The drawing under review shows one solid part. Ordinate dimensions are in mm from its lowest x, y, z. A direction names the side the tool comes from. Give positions to 0.01 mm unless a question says otherwise; leave off trailing zeros. Write each loop counter-clockwise with the first axis right and the second up, starting at its lowest first coordinate (ties: lowest second). Pieces come first, ordered by that corner, then holes. Notation, with made-up numbers: (69, -7.5) - (76, -7.5) arc R25 ccw to (76, 22.5) - close; hole circle Ø10 at (-1.75, -9). An arc over 180 degrees is marked (long way). Write each question's results on one line, items separated by ' | '. Start each with the question number.
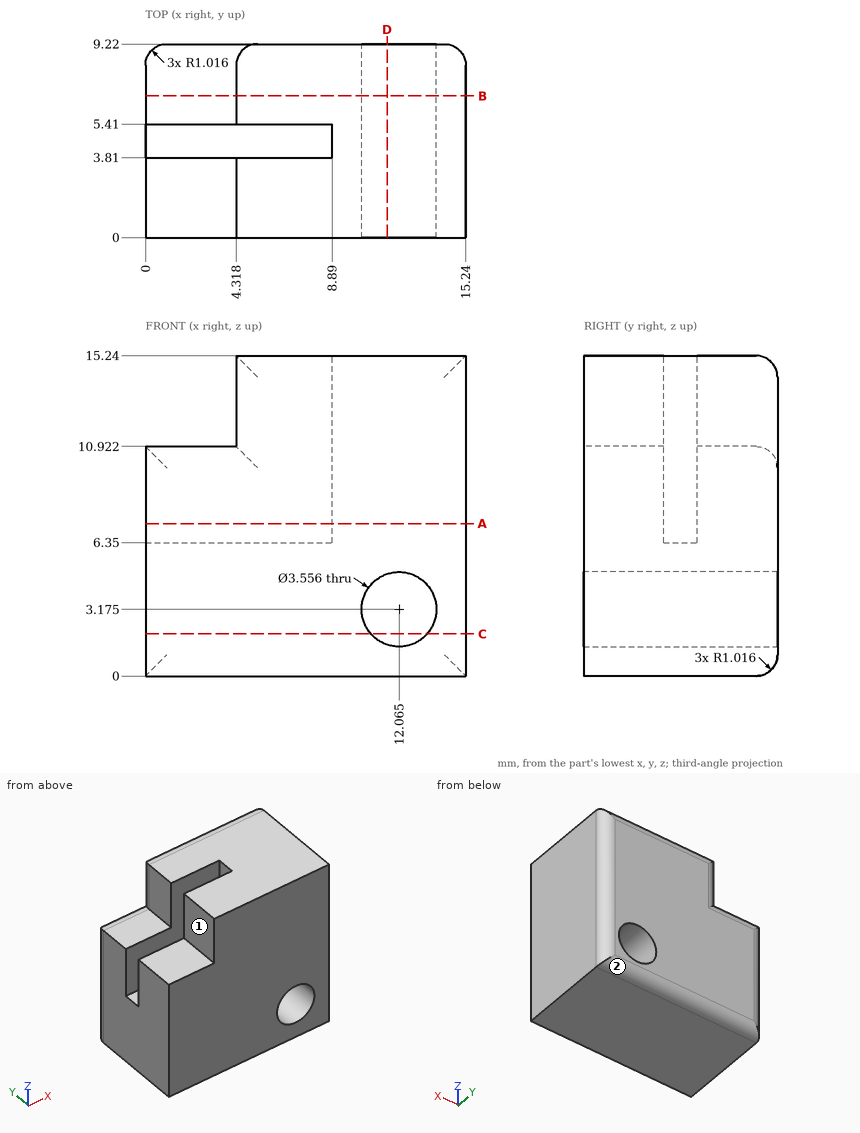
Q1. Add section D-D on x = 11.5. State the section outline as (y, z) points, plus the area to 3 significant figures.
Q2. Machinability: for the marked faces 1 and 2, which of the approach directions +Z, -Z, +X, -X, +Y, -Y give a long, thin tool a straight path to every point of the face, cutting with its end or side? Answer none if there is none.
Q3. Add section A-A on z = 7.25. State the section outline as (x, y) points.
Q4. Insertion check: P1, Ø3, axis at y = 2.5, z = 14, coming from the -X side; P2, Ø0.8, axis at y = 4.5, z = 13, coming from the -X side; P3, Ø0.8, axis at x = 3, y = 4.5, coming from the +Z side. Each pin has a flat end and moves straight along its axis. Give the tip position at first contact, or say it passes through.
Q5. Add section B-B on y = 6.75. State the section outline as (x, z) points (3 decimals), plus the area to 3 significant figures.
Q6. For line 1 along Y through (x, z) = (8, 14.25); line 2 along X through (y, z) = (1.75, 3.25); line 3 along Z through (x, y) = (4.5, 5), list the stretches that pass through material, from the lowest coordinate up. Write a range as [from, to].
Q7. Add section C-C on z = 2. State the section outline as (x, y) points.
Result:
1) outline: (0, 0) - (8.2, 0) arc R1.02 ccw to (9.22, 1.02) - (9.22, 1.49) - (0, 1.49) - close; (0, 4.86) - (9.22, 4.86) - (9.22, 14.22) arc R1.02 ccw to (8.2, 15.24) - (0, 15.24) - close | area: 109 mm²
2) face 1: +Z, -X, +Y, -Y | face 2: -Z, +X, -X, +Y
3) outline: (0, 0) - (15.24, 0) - (15.24, 8.2) arc R1.02 ccw to (14.22, 9.22) - (1.02, 9.22) arc R1.02 ccw to (0, 8.2) - (0, 5.41) - (8.89, 5.41) - (8.89, 3.81) - (0, 3.81) - close
4) P1: stops at x = 4.32 | P2: stops at x = 8.89 | P3: stops at z = 6.35
5) outline: (0, 0) - (15.24, 0) - (15.24, 15.24) - (4.318, 15.24) - (4.318, 10.922) - (0, 10.922) - close; hole circle Ø3.556 at (12.065, 3.175) | area: 204 mm²
6) line 1: y = [0, 3.81], [5.41, 9.22] | line 2: x = [0, 10.29], [13.84, 15.24] | line 3: z = [0, 6.35]
7) outline: (0, 0) - (10.73, 0) - (10.73, 9.22) - (1.02, 9.22) arc R1.02 ccw to (0, 8.2) - close; (13.4, 0) - (15.24, 0) - (15.24, 8.2) arc R1.02 ccw to (14.22, 9.22) - (13.4, 9.22) - close
